```python
from build123d import *

# Parameters (mm, degrees)
F2_R     = 242.5
F2_R_2   = 12.7
F2_R_3   = 190.5
F4_DEPTH = 30.2
F5_DEPTH = 31.8


with BuildPart() as f4:
    # F2 (on Top) → F4 (new body)
    with BuildSketch(Plane.XY):
        Circle(F2_R)
        with Locations((-152.6643540582, -152.6643540582)):
            Circle(F2_R_2, mode=Mode.SUBTRACT)
        with Locations((-55.8790318376, -208.5433858958)):
            Circle(F2_R_2, mode=Mode.SUBTRACT)
        with Locations((-208.5433858958, -55.8790318376)):
            Circle(F2_R_2, mode=Mode.SUBTRACT)
        with Locations((55.8790318376, -208.5433858958)):
            Circle(F2_R_2, mode=Mode.SUBTRACT)
        with Locations((152.6643540582, -152.6643540582)):
            Circle(F2_R_2, mode=Mode.SUBTRACT)
        with Locations((208.5433858958, -55.8790318376)):
            Circle(F2_R_2, mode=Mode.SUBTRACT)
        with Locations((-208.5433858958, 55.8790318376)):
            Circle(F2_R_2, mode=Mode.SUBTRACT)
        with Locations((-152.6643540582, 152.6643540582)):
            Circle(F2_R_2, mode=Mode.SUBTRACT)
        with Locations((-55.8790318376, 208.5433858958)):
            Circle(F2_R_2, mode=Mode.SUBTRACT)
        Circle(F2_R_3, mode=Mode.SUBTRACT)
        with Locations((208.5433858958, 55.8790318376)):
            Circle(F2_R_2, mode=Mode.SUBTRACT)
        with Locations((55.8790318376, 208.5433858958)):
            Circle(F2_R_2, mode=Mode.SUBTRACT)
        with Locations((152.6643540582, 152.6643540582)):
            Circle(F2_R_2, mode=Mode.SUBTRACT)
    extrude(amount=F4_DEPTH)

    # F3 (on face) → F5 (join)
    with BuildSketch(Plane.XY):
        with BuildLine():
            Line((-100, -162.1426840779), (-100, -161.554944214))
            ThreePointArc((-100, -161.554944214), (0, -190), (100, -161.554944214))
            Line((100, -161.554944214), (100, -162.1426840779))
            ThreePointArc((100, -162.1426840779), (166.3433948193, -92.8446282776), (190.5, 0))
            ThreePointArc((190.5, 0), (-92.8446282776, 166.3433948193), (-100, -162.1426840779))
        make_face()
    extrude(amount=F5_DEPTH)


solid = f4.part
```
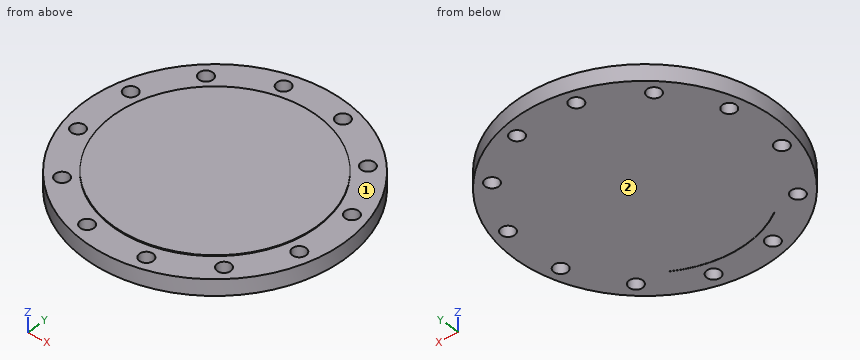
CAD build for the part. Positions are in the model's coordinates, mm. Face numbers are marked on the shaded views. A direction names the side the tool comes from. Round coordinates to 2 decimals unless told otherwise and drop trailing zeros. Order: outer loops, then holes, each group sorted by start corner. A loop starts at its lowest first (then second) coordinate and runs counter-clockwise, first axis right, second up. Notation, with made-up numbers: (54, 65.5) - (106, 65.5) arc R19 cw to (106, 90.5) - close; hole circle Ø8 at (81, 8). An arc over 180 degrees is marked (long way). Answer in a Markdown table with one row per item. Add a question column.
(1) Band-saw the part on D-D on x = -171.5. List the corners of the cut face in (y, z).
(2) Band-saw the part on B-B on x = -89. List the corners of the cut face in (y, z).
(3) Drop flat-ended pins along their axis: pin 1 Ø0.6 at (y, z) = (-162, 19.5) entering from -X; pin 2 Ø10 at (y, z) = (-178.5, 27.5) entering from -X; pin 3 Ø1.5 at (y, z) = (46.5, 12) entering from -X. Give the stop position or say it passes through.
(4) 3-axis set-ups, long thin cutter, end or side, ignore diameter. For the marked faces 1 and 2: which of +Z, -Z, +X, -X, +Y, -Y reach the whole face in a straight line?
(5) Band-saw the part on A-A on z = 7. Count the separate pieces of the cut face and the enclosed holes in it, and give its area (3 significant figures).
(6) Probe L1, parallel to X at y = -172.5, z = 11.5; L2, parallel to X at y = -212, z = 21; L3, parallel to Y at x = -149, z = 8. List the from-to ranges inside material, lowest first. Write a range as [from, to].
(7) Band-saw the part on C-C on y = 147. List the corners of the cut face in (x, z).
Data:
| question | item | result |
|---|---|---|
| 1 | outline | (-171.45, 0) - (171.45, 0) - (171.45, 30.2) - (82.93, 30.2) - (82.93, 31.8) - (-82.93, 31.8) - (-82.93, 30.2) - (-171.45, 30.2) - close |
| 2 | outline | (-225.58, 0) - (-168.43, 0) - (-168.43, 30.2) - (-225.58, 30.2) - close; (-167.87, 0) - (225.58, 0) - (225.58, 30.2) - (168.43, 30.2) - (168.43, 31.8) - (-167.87, 31.8) - close |
| 3 | pin 1 | stops at x = -180.72 |
| 3 | pin 2 | stops at x = -169.42 |
| 3 | pin 3 | stops at x = -238.15 |
| 4 | face 1 | +Z |
| 4 | face 2 | -Z, +X, -X, +Y, -Y |
| 5 | separate pieces | 1 |
| 5 | enclosed holes | 13 |
| 5 | area | 179,000 mm^2 |
| 6 | L1 | x = [-170.44, -80.83], [-79.65, 79.65], [80.83, 170.44] |
| 6 | L2 | x = [-117.74, -68.1], [-43.66, 43.66], [68.1, 117.74] |
| 6 | L3 | y = [-191.32, -164.82], [-140.5, 140.5], [164.82, 191.32] |
| 7 | outline | (-192.87, 0) - (-164.03, 0) - (-164.03, 30.2) - (-192.87, 30.2) - close; (-141.3, 0) - (141.3, 0) - (141.3, 30.2) - (121.17, 30.2) - (121.17, 31.8) - (-121.17, 31.8) - (-121.17, 30.2) - (-141.3, 30.2) - close; (164.03, 0) - (192.87, 0) - (192.87, 30.2) - (164.03, 30.2) - close |
